Build history of the part. All positions in model axes, mm. A direction names the side the tool comes from. Give positions to 0.01 mm unless a question says otherwise; leave off trailing zeros. Write each loop counter-clockwise with the first axis right and the second up, starting at its lowest first coordinate (ties: lowest second). Pieces come first, ordered by that corner, then holes. Notation, with made-up numbers: (19, -8) -> (41, -8) arc R8 cw to (41, 5) -> close; hole circle Ø10 at (-23, -8.75). An arc over 180 degrees is marked (long way). One line per question, with ' | ' between items. Start each with the question number.
(1) Tool access for faces 1 (the flat face through (0, 2, -2)), 2 (the flat face through (0, -18, 0)): list every direction of +Z, -Z, +X, -X, +Y, -Y with a clear straight run to the whole face (end or side of a thin tool).
(2) Band-saw the part on C-C, the plane y = -15.5. Give the cut face in (x, z).
(3) Band-saw the part on A-A, the plane z = 0. Give the cut face in (x, y), and give its area (4 significant figures).
(4) Band-saw the part on B-B, the plane x = 0. Give the cut face in (y, z), and give its area (4 significant figures).
(5) Drill centre lines: probe 1 along Z at (x, y) = (0, -9.75) (3 decimals); probe 2 along Z at (x, y) = (0, -11.25); probe 3 along Z at (x, y) = (7.25, -6.25). Where is each one in solid material? Low to high. Write a range as from..to.
(6) Band-saw the part on D-D, the plane y = -19.25. Give the cut face in (x, z), and give its area (3 significant figures).
(7) Pull direction Z, two halves, no side cores. Call faces 3 (the cylindrical face through (1.5, -7.86, 0.07)), 4 (the cylindrical face through (-7.62, 0.99, -3.16)), 5 (the flat face through (0, -25.5, 0)): released by +Z, released by -Z, zero draft, split by the parting line, or undercut.
(8) Pin check, flat tips, straight feed: P1, Ø1.5, axis at x = -0.5, y = -19, coming from the +Z side; P2, Ø5, axis at x = -1, y = -7.5, coming from the +Z side; P3, Ø8, axis at x = 0.5, y = -17, coming from the -Z side. Stop position of each tip, or through.
from build123d import *

# Parameters (mm, degrees)
F0_R     = 12
F1_DEPTH = 25.5
F3_R     = 2
F4_R     = 8.25
F5_DEPTH = 2
F6_R     = 1.5
F7_DEPTH = 20


# Not quite as in the source:
# - a fillet or chamfer that OpenCascade refuses, or shapes differently, is made with other operations: its cross-section is extruded or revolved along the edge and cut away or added


with BuildPart() as f1:
    # F0 (on Front) → F1 (new body)
    with BuildSketch(Plane.XZ):
        Circle(F0_R)
    extrude(amount=F1_DEPTH)

    # F2: chamfer of 5.5 x 35 on 1 edges, made by hand

    # F2_s1 → F2_t2 (revolve, cut)
    with BuildSketch(Plane.XY):
        Polygon((12, 9.5), (6.5, -25.5), (12, -25.5), align=None)
    revolve(axis=Axis((0, -25.5, 0), (0, -1, 0)), mode=Mode.SUBTRACT)

    # F3
    f3_edges = [f1.edges().sort_by_distance(p)[0] for p in [
        (-6.5, -25.5, 0),
    ]]
    fillet(f3_edges, radius=F3_R)

    # F4 (on face) → F5 (join)
    with BuildSketch(Plane(origin=(0, 0, 0), x_dir=(-1, 0, 0), z_dir=(0, 1, 0))):
        Circle(F4_R)
    extrude(amount=F5_DEPTH)

    # F6 (on face) → F7 (cut)
    with BuildSketch(Plane(origin=(0, 2, 0), x_dir=(-1, 0, 0), z_dir=(0, 1, 0))):
        Circle(F6_R)
    extrude(amount=-F7_DEPTH, mode=Mode.SUBTRACT)


solid = f1.part
Results:
1) face 1: +Z, -Z, +X, -X, +Y | face 2: +Y
2) outline: circle Ø16.14 at (0, 0); hole circle Ø3 at (0, 0)
3) outline: (-10.51, 0) -> (-6.77, -23.81) arc R2 ccw to (-4.79, -25.5) -> (4.79, -25.5) arc R2 ccw to (6.77, -23.81) -> (10.51, 0) -> (8.25, 0) -> (8.25, 2) -> (1.5, 2) -> (1.5, -18) -> (-1.5, -18) -> (-1.5, 2) -> (-8.25, 2) -> (-8.25, 0) -> close | area: 405.5 mm²
4) outline: (-25.5, -4.79) arc R2 ccw to (-23.81, -6.77) -> (0, -10.51) -> (0, -8.25) -> (2, -8.25) -> (2, -1.5) -> (-18, -1.5) -> (-18, 1.5) -> (2, 1.5) -> (2, 8.25) -> (0, 8.25) -> (0, 10.51) -> (-23.81, 6.77) arc R2 ccw to (-25.5, 4.79) -> close | area: 405.5 mm²
5) probe 1: z = -8.975..-1.5, 1.5..8.975 | probe 2: z = -8.74..-1.5, 1.5..8.74 | probe 3: z = -6.18..6.18
6) outline: circle Ø14.96 at (0, 0) | area: 176 mm²
7) face 3: undercut | face 4: split by the parting line | face 5: zero draft
8) P1: stops at z = 7.63 | P2: stops at z = 9.7 | P3: stops at z = -8.46
